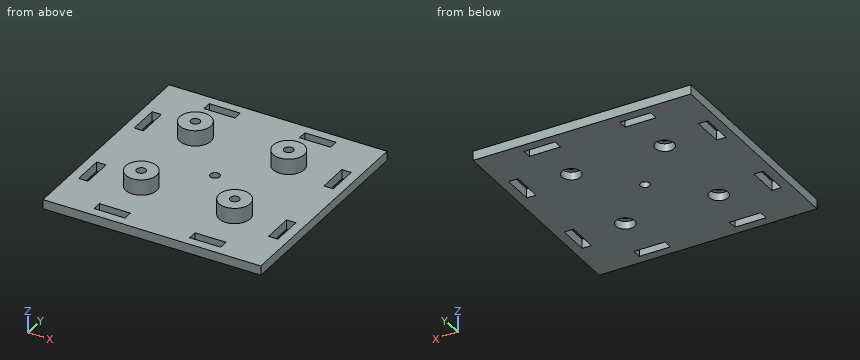
from build123d import *

# Parameters (mm, degrees)
SKETCH_W                 = 70
SKETCH_H                 = 70
EXTRUDE_DEPTH            = 3
SKETCH001_R              = 5
PAD_DEPTH                = 5
POLARPATTERN_COUNT       = 4
SKETCH002_R              = 1.5
POCKET_DEPTH             = 206.636344
POLARPATTERN001_COUNT    = 4
SKETCH003_R              = 3
POCKET001_DEPTH          = 2.5
POLARPATTERN002_COUNT    = 4
SKETCH004_W              = 10
SKETCH004_H              = 3
POCKET002_DEPTH          = 5
POLARPATTERN002002_COUNT = 4
SKETCH005_R              = 1.5
POCKET003_DEPTH          = 8.001


with BuildPart() as part:
    # Sketch → Extrude (new body)
    with BuildSketch(Plane.XY):
        Rectangle(SKETCH_W, SKETCH_H)
    extrude(amount=EXTRUDE_DEPTH)

    # Sketch001 → Pad (new body)
    with BuildSketch(Plane.XY.offset(3)):
        with Locations((-15, 15)):
            Circle(SKETCH001_R)
    pad = extrude(amount=PAD_DEPTH)

    # PolarPattern: Pad ×4 about axis
    polarpattern_axis = Axis((0, 0, 3), (0, 0, 1))
    for i in range(1, POLARPATTERN_COUNT):
        add(pad.rotate(polarpattern_axis, i * 360 / POLARPATTERN_COUNT))

    # Sketch002 → Pocket (cut, through all)
    with BuildSketch(Plane.XY.offset(8)):
        with Locations((-15, 15)):
            Circle(SKETCH002_R)
    pocket = extrude(amount=-POCKET_DEPTH, mode=Mode.SUBTRACT)

    # PolarPattern001: Pocket ×4 about axis
    polarpattern001_axis = Axis((0, 0, 8), (0, 0, 1))
    for i in range(1, POLARPATTERN001_COUNT):
        add(pocket.rotate(polarpattern001_axis, i * 360 / POLARPATTERN001_COUNT), mode=Mode.SUBTRACT)

    # Sketch003 → Pocket001 (cut)
    with BuildSketch(Plane(origin=(0, 0, 0), x_dir=(1, 0, 0), z_dir=(0, 0, -1))):
        with Locations((-15, 15)):
            Circle(SKETCH003_R)
    pocket001 = extrude(amount=-POCKET001_DEPTH, mode=Mode.SUBTRACT)

    # PolarPattern002: Pocket001 ×4 about axis
    polarpattern002_axis = Axis((0, 0, 0), (0, 0, -1))
    for i in range(1, POLARPATTERN002_COUNT):
        add(pocket001.rotate(polarpattern002_axis, i * 360 / POLARPATTERN002_COUNT), mode=Mode.SUBTRACT)

    # Sketch004 → Pocket002 (cut)
    with BuildSketch(Plane(origin=(0, 0, 0), x_dir=(1, 0, 0), z_dir=(0, 0, -1))):
        with Locations((15.374485, 30.5)):
            Rectangle(SKETCH004_W, SKETCH004_H)
        with Locations((-15.374485, 30.5)):
            Rectangle(SKETCH004_W, SKETCH004_H)
    pocket002 = extrude(amount=-POCKET002_DEPTH, mode=Mode.SUBTRACT)

    # PolarPattern002002: Pocket002 ×4 about axis
    polarpattern002002_axis = Axis((0, 0, 0), (0, 0, -1))
    for i in range(1, POLARPATTERN002002_COUNT):
        add(pocket002.rotate(polarpattern002002_axis, i * 360 / POLARPATTERN002002_COUNT), mode=Mode.SUBTRACT)

    # Sketch005 → Pocket003 (cut, through all)
    with BuildSketch(Plane(origin=(0, 0, 0), x_dir=(1, 0, 0), z_dir=(0, 0, -1))):
        Circle(SKETCH005_R)
    extrude(amount=-POCKET003_DEPTH, mode=Mode.SUBTRACT)


solid = part.part
Build history of the part. All positions in model axes, mm. Round coordinates to 2 decimals unless told otherwise and drop trailing zeros. Write each loop counter-clockwise with the first axis right and the second up, starting at its lowest first coordinate (ties: lowest second). Pieces come first, ordered by that corner, then holes. Notation, with made-up numbers: (-22.75, 62.5) -> (12.25, 62.5) arc R21 ccw to (12.25, 75.5) -> close; hole circle Ø2 at (69.5, 15). An arc over 180 degrees is marked (long way). Use one line per item in the form item = value.
Q1. Band-saw the part on A-A, the plane z = 5. Write the cut outline in (x, y).
Conclusion:
outline = circle Ø10 at (-15, -15); circle Ø10 at (-15, 15); circle Ø10 at (15, -15); circle Ø10 at (15, 15); hole circle Ø3 at (-15, -15); hole circle Ø3 at (-15, 15); hole circle Ø3 at (15, -15); hole circle Ø3 at (15, 15)
Q2. Band-saw the part on D-D, the plane y = -15. State how many separate pieces and enclosed holes the cut face has, then the cut area to 3 significant figures.
Conclusion:
separate_pieces = 5
enclosed_holes = 0
area = 229 mm²
Q3. Drill centre lines: L1, parallel to X at y = -15, z = 4.7; L2, parallel to Y at x = -15, z = 1.1. Where is each one in solid material? Low to high.
Conclusion:
L1 = -20 to -16.5, -13.5 to -10, 10 to 13.5, 16.5 to 20
L2 = -35 to -32, -29 to -18, -12 to 12, 18 to 29, 32 to 35
Q4. Drop flat-ended pins along their axis: P1, Ø2, axis at x = 16, z = 6.5, coming from the -Y side; P2, Ø4, axis at x = 0, y = 0, coming from the +Z side; P3, Ø3, axis at x = 15, y = -15.5, coming from the -Z side. Give the stop position or say it passes through.
Conclusion:
P1 = -20
P2 = 3
P3 = 2.5
Q5. Band-saw the part on B-B, the plane y = 0. Write the cut outline in (x, z).
Conclusion:
outline = (-35, 0) -> (-1.5, 0) -> (-1.5, 3) -> (-35, 3) -> close; (1.5, 0) -> (35, 0) -> (35, 3) -> (1.5, 3) -> close
